Geometry: final body of the model. Coordinates: model frame, mm. Face numbers are marked on the shaded views. A direction names the side the tool comes from. Give positions to 0.01 mm unless a question says otherwise; leave off trailing zeros. Order: outer loops, then holes, each group sorted by start corner. A loop starts at its lowest first (then second) coordinate and runs counter-clockwise, first axis right, second up. Notation, with made-up numbers: (69.25, 34.5) - (103.25, 34.5) arc R11 cw to (103.25, 50.5) - close; hole circle Ø8 at (57, 72). An arc over 180 degrees is marked (long way). One line per item, written item: value.
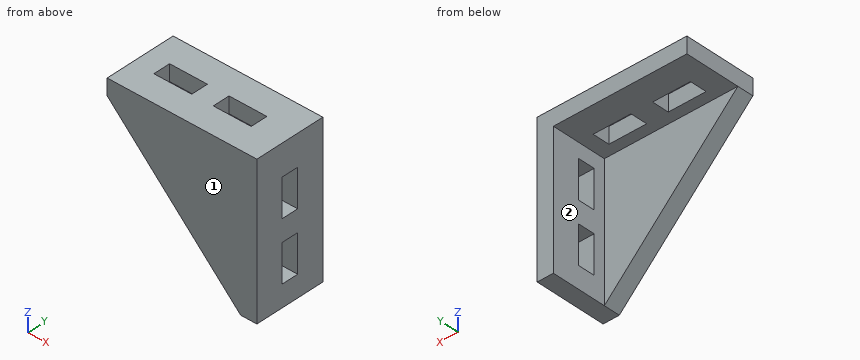
```python
from build123d import *

# Parameters (mm, degrees)
BOSS_EXTRUDE1_DEPTH = 42
BOSS_EXTRUDE2_DEPTH = 9.525
SKETCH3_W           = 22.225
SKETCH3_H           = 10
CUT_EXTRUDE1_DEPTH  = 9.525
SKETCH4_W           = 22.225
SKETCH4_H           = 10
CUT_EXTRUDE2_DEPTH  = 9.525


with BuildPart() as part:
    # Sketch1 → Boss-Extrude1 (new body)
    with BuildSketch(Plane(origin=(0, 0, 0), x_dir=(1, 0, 0), z_dir=(0, 1, 0))):
        Polygon((0, 0), (-88, 0), (-88, 9.525), (-9.525, 9.525), (-9.525, 88), (0, 88), align=None)
    extrude(amount=BOSS_EXTRUDE1_DEPTH)

    # Sketch2 → Boss-Extrude2 (add)
    with BuildSketch(Plane(origin=(0, 0, 0), x_dir=(1, 0, 0), z_dir=(0, 1, 0))):
        Polygon((-9.525, 88), (-88, 9.525), (-9.525, 9.525), align=None)
    extrude(amount=BOSS_EXTRUDE2_DEPTH)

    # Sketch3 → Cut-Extrude1 (cut)
    with BuildSketch(Plane(origin=(0, 0, -9.525), x_dir=(-1, 0, 0), z_dir=(0, 0, -1))):
        with Locations((29.2625, 21)):
            Rectangle(SKETCH3_W, SKETCH3_H)
        with Locations((64.1875, 21)):
            Rectangle(SKETCH3_W, SKETCH3_H)
    extrude(amount=-CUT_EXTRUDE1_DEPTH, mode=Mode.SUBTRACT)

    # Sketch4 → Cut-Extrude2 (cut)
    with BuildSketch(Plane.ZY.offset(9.525)):
        with Locations((-29.2625, 21)):
            Rectangle(SKETCH4_W, SKETCH4_H)
        with Locations((-64.1875, 21)):
            Rectangle(SKETCH4_W, SKETCH4_H)
    extrude(amount=-CUT_EXTRUDE2_DEPTH, mode=Mode.SUBTRACT)


solid = part.part
```
1) Section C-C, the plane x = -59. Return loops of the section in (y, z) (3 decimals), then the cut area to 3 significant figures.
Answers below:
outline: (0, -38.525) - (9.525, -38.525) - (9.525, -9.525) - (16, -9.525) - (16, 0) - (0, 0) - close; (26, -9.525) - (42, -9.525) - (42, 0) - (26, 0) - close
area: 581 mm^2
2) First-contact query: pin 1 (6 mm diameter, centred on x = -16.5, z = -35.5, fed in from +Y) (3 decimals); pin 2 (16 mm diameter, centred on x = -31, y = 18.5, fed in from -Z) (3 decimals); pin 3 (2 mm diameter, centred on y = 8.5, z = -59, fed in from -X) (3 decimals). Flat tips, straight axial feed; report the tip coordinate or a pass-through.
Answers below:
pin 1: y = 9.525
pin 2: z = -9.525
pin 3: x = -39.525
3) Section B-B, the plane z = -8. Return loops of the section in (x, y) (3 decimals), then the cut area to 3 significant figures.
Answers below:
outline: (-88, 0) - (0, 0) - (0, 42) - (-88, 42) - close; hole (-75.3, 16) - (-53.075, 16) - (-53.075, 26) - (-75.3, 26) - close; hole (-40.375, 16) - (-18.15, 16) - (-18.15, 26) - (-40.375, 26) - close
area: 3,250 mm^2
4) Section D-D, the plane z = -65.5. Return loops of the section in (x, y) (3 decimals).
Answers below:
outline: (-32.025, 0) - (0, 0) - (0, 16) - (-9.525, 16) - (-9.525, 9.525) - (-32.025, 9.525) - close; (-9.525, 26) - (0, 26) - (0, 42) - (-9.525, 42) - close
5) Material intervals for line 1 along Z through (x, y) = (-8, 20) (3 decimals); line 2 along X through (y, z) = (12.5, -46) (3 decimals), sorted ascending.
Answers below:
line 1: -88 to -75.3, -53.075 to -40.375, -18.15 to 0
line 2: -9.525 to 0
6) Section A-A, the plane y = 18.5. Return loops of the section in (x, z) (3 decimals), then the cut area to 3 significant figures.
Answers below:
outline: (-88, -9.525) - (-75.3, -9.525) - (-75.3, 0) - (-88, 0) - close; (-53.075, -9.525) - (-40.375, -9.525) - (-40.375, 0) - (-53.075, 0) - close; (-18.15, -9.525) - (-9.525, -9.525) - (-9.525, -18.15) - (0, -18.15) - (0, 0) - (-18.15, 0) - close; (-9.525, -88) - (0, -88) - (0, -75.3) - (-9.525, -75.3) - close; (-9.525, -53.075) - (0, -53.075) - (0, -40.375) - (-9.525, -40.375) - close
area: 739 mm^2
7) Set-up query: the marked faces 1 and 2. Return all of +Z, -Z, +X, -X, +Y, -Y with unobstructed straight access to the full face (end or side cutting, diameter ignored); none if empty.
Answers below:
face 1: +Z, -Z, +X, -X, -Y
face 2: -Z, -X, +Y
